Drawing for the job (mm, zero at the part's lowest x, y, z). Round coordinates to 2 decimals unless told otherwise and drop trailing zeros. Loops run counter-clockwise (first coordinate to the right, second up) from the corner with the lowest first, then second, coordinate; pieces in that order, holes last. Notation, with made-up numbers: (55.25, -8) -> (86.25, -8) arc R5 ccw to (86.25, 1) -> close; hole circle Ø1 at (19.5, 15). An arc over 180 degrees is marked (long way). Put each result on its own line as item: value. Start each with the question number.
Item 1: Flat gauge pin, fed straight in: pin 1 Ø8.5 at (x, z) = (114.3, 114.3) entering from +Y (1 decimal). Where does the tip first touch, or does it go through?
Item 2: Cut at D-D, the plane x = 54. List the corners of the cut face in (y, z) (1 decimal).
Item 3: Cut at B-B, the plane z = 63.5. List the corners of the cut face in (x, y) (1 decimal).
Item 4: Cut at C-C, the plane x = 35.12. List the corners of the cut face in (y, z) (1 decimal), plus the area to 3 significant figures.
Item 5: Cut at A-A, the plane z = 44. List the corners of the cut face in (x, y) (1 decimal), plus the area to 3 significant figures.
Item 6: Drill centre lines: probe 1 along Z at (x, y) = (114, 2); probe 2 along Z at (x, y) = (91.88, 1.55) (1 decimal); probe 3 along X at (y, z) = (1.15, 63.5) (1 decimal). Where is each one in solid material? Low to high. Write a range as [from, to].
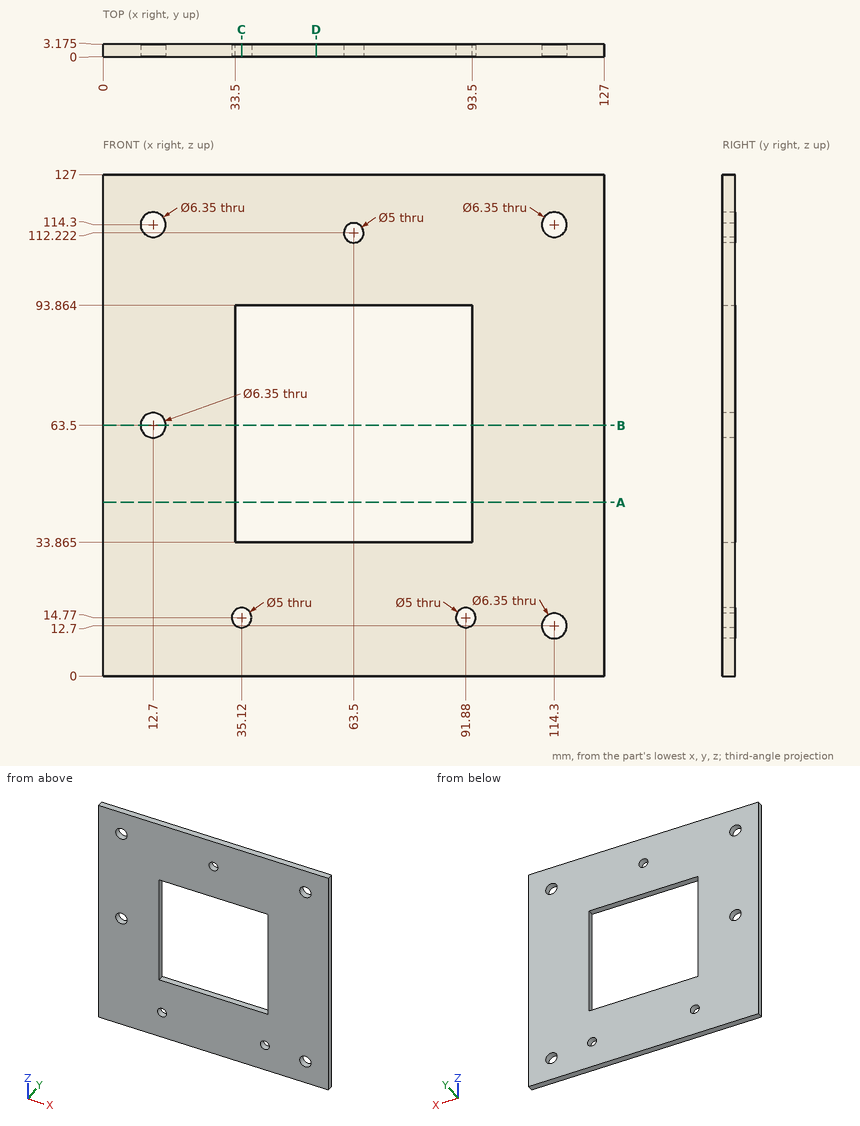
Reply:
1. pin 1: stops at y = 3.2
2. outline: (0, 0) -> (3.2, 0) -> (3.2, 33.9) -> (0, 33.9) -> close; (0, 93.9) -> (3.2, 93.9) -> (3.2, 127) -> (0, 127) -> close
3. outline: (0, 0) -> (9.5, 0) -> (9.5, 3.2) -> (0, 3.2) -> close; (15.9, 0) -> (33.5, 0) -> (33.5, 3.2) -> (15.9, 3.2) -> close; (93.5, 0) -> (127, 0) -> (127, 3.2) -> (93.5, 3.2) -> close
4. outline: (0, 0) -> (3.2, 0) -> (3.2, 12.3) -> (0, 12.3) -> close; (0, 17.3) -> (3.2, 17.3) -> (3.2, 33.9) -> (0, 33.9) -> close; (0, 93.9) -> (3.2, 93.9) -> (3.2, 127) -> (0, 127) -> close
4. area: 197 mm^2
5. outline: (0, 0) -> (33.5, 0) -> (33.5, 3.2) -> (0, 3.2) -> close; (93.5, 0) -> (127, 0) -> (127, 3.2) -> (93.5, 3.2) -> close
5. area: 213 mm^2
6. probe 1: z = [0, 9.54], [15.86, 111.14], [117.46, 127]
6. probe 2: z = [0, 12.3], [17.3, 33.9], [93.9, 127]
6. probe 3: x = [0, 9.5], [15.9, 33.5], [93.5, 127]
